Geometry check sheet. Reference: the model listing, model coordinates, mm. Round coordinates to 2 decimals unless told otherwise and drop trailing zeros. Order: outer loops, then holes, each group sorted by start corner. A loop starts at its lowest first (then second) coordinate and runs counter-clockwise, first axis right, second up. Notation, with made-up numbers: (85.25, 17) - (118.25, 17) arc R16 ccw to (118.25, 39) - close; hole circle Ø2 at (73.25, 57.25). An arc over 180 degrees is marked (long way). Return JSON: item names as keys, results as strings. Group by question number.
Q1. Gauge pin test, flat ends, axial feed: pin 1 Ø1.5 at (x, z) = (-5, -2) entering from +Y; pin 2 Ø3 at (x, z) = (-4.5, -1.5) entering from -Y; pin 3 Ø8.5 at (x, y) = (0, 0) entering from -Z. Record the tip position at first contact, or that the pin passes through.
Q2. Material ranges on line 1 along X through (y, z) = (-3, -0.85); line 2 along Y through (x, z) = (1, -2.65); line 3 along X through (y, z) = (-0.5, -1.9), recorded low to high.
Q3. Sectioned sample at A-A, the plane z = -2.7. Record the cut outline in (x, y).
Q4. Draft check along Y on faces 1 (the cylindrical face through (-0.86, -3.874, -2.903)), 2 (the conical face through (0.018, -7.406, -0.232)), 3 (the conical face through (6.4, 3.72, -0.23)). Enter one of: pulls with the +Y half, pulls with the -Y half, needs draft (parallel to the pull), parting line crosses it, or undercut.
```python
from build123d import *

# Parameters (mm, degrees)
THREADSCHEMATIC_START     = -5.7658
THREADSCHEMATIC_OUTLINE_R = 3.96875
THREADSCHEMATIC_DEPTH     = 5.7658


# Read off the part's stored shape, not the designer's step: ThreadSchematic
with BuildPart() as part:
    # ThreadSchematic outline → ThreadSchematic (new body)
    with BuildSketch(Plane.XY.offset(THREADSCHEMATIC_START)):
        Polygon((7.1374, 4.120779811), (0, 8.241559623), (-7.1374, 4.120779811), (-7.1374, -4.120779811), (0, -8.241559623), (7.1374, -4.120779811), align=None)
        Circle(THREADSCHEMATIC_OUTLINE_R, mode=Mode.SUBTRACT)
    extrude(amount=THREADSCHEMATIC_DEPTH)

    # Sketch3 → Double-Chamfer (revolve, cut)
    with BuildSketch(Plane(origin=(0, 0, 0), x_dir=(0, 0, -1), z_dir=(1, 0, 0))):
        Polygon((5.7658, 7.1374), (4.8133, 8.241559623), (4.8133, 20.941559623), (18.4658, 20.941559623), (18.4658, 7.1374), align=None)
        Polygon((0.9525, 20.941559623), (-12.7, 20.941559623), (-12.7, 7.1374), (0, 7.1374), (0.9525, 8.241559623), align=None)
    revolve(axis=Axis((0, 0, 0), (0, 0, -1)), mode=Mode.SUBTRACT)

    # EndChamferSke → EndChamfer (revolve, cut)
    with BuildSketch(Plane(origin=(0, 0, 0), x_dir=(0, 0, -1), z_dir=(1, 0, 0)), mode=Mode.PRIVATE) as endchamfer_sk:
        Polygon((5.7404, 4.7625), (5.129031293, 3.889375), (5.7912, 3.889375), (5.7912, 4.7625), align=None)
        Polygon((-0.0508, 4.7625), (0, 4.7625), (0.611368707, 3.889375), (-0.0508, 3.889375), align=None)
    revolve(endchamfer_sk.sketch.rotate(Axis((0, 0, -25.037505729), (0, 0, -1)), 90), axis=Axis((0, 0, -25.037505729), (0, 0, -1)), mode=Mode.SUBTRACT)


solid = part.part
```
Reply:
{
 "1": {"pin 1": "y = 5.79", "pin 2": "y = -6.51", "pin 3": "z = -5.38"},
 "2": {"line 1": "-7.14 to -2.6, 2.6 to 7.14", "line 2": "-7.66 to -3.84, 3.84 to 7.66", "line 3": "-7.14 to -3.94, 3.94 to 7.14"},
 "3": {"outline": "(-7.14, -4.12) - (0, -8.24) - (7.14, -4.12) - (7.14, 4.12) - (0, 8.24) - (-7.14, 4.12) - close; hole circle Ø7.94 at (0, 0)"},
 "4": {"face 1": "undercut", "face 2": "pulls with the -Y half", "face 3": "pulls with the +Y half"}
}
